```python
from build123d import *

# Parameters (mm, degrees)
SKETCH_1_W      = 10
SKETCH_1_H      = 40
SKETCH_1_W_2    = 40
SKETCH_1_H_2    = 10
EXTRUDE_1_DEPTH = 160


with BuildPart() as part:
    # Sketch 1 → Extrude 1 (new body)
    with BuildSketch(Plane.XY):
        Polygon((-25, 20), (-5, 20), (5, 20), (25, 20), (25, 30), (-25, 30), align=None)
        Rectangle(SKETCH_1_W, SKETCH_1_H)
        Polygon((5, -20), (-5, -20), (-30, -20), (-30, -30), (-20, -30), (20, -30), (30, -30), (30, -20), align=None)
        with Locations((0, -35)):
            Rectangle(SKETCH_1_W_2, SKETCH_1_H_2)
    extrude(amount=EXTRUDE_1_DEPTH)


solid = part.part
```
Could you check a few things on this model? Use its own coordinates, in mm. A direction names the side the tool comes from. Give positions to 0.01 mm unless a question says otherwise; leave off trailing zeros. Loops run counter-clockwise (first coordinate to the right, second up) from the corner with the lowest first, then second, coordinate; pieces in that order, holes last. Notation, with made-up numbers: (88.25, 79.5) - (106.25, 79.5) arc R25 cw to (106.25, 109.5) - close; hole circle Ø10 at (21.5, 9). An arc over 180 degrees is marked (long way). Use one line per item in the form item = value.
1. I want a section at D-D (y = 16). Please give me the cut outline in (x, z).
Response values:
outline = (-5, 0) - (5, 0) - (5, 160) - (-5, 160) - close
2. I need wall thicknesses on probe 1 along Y at (x, z) = (18, 16); probe 2 along Y at (x, z) = (23, 23); probe 3 along X at (y, z) = (-9, 140). Which ranges of each line are inside material? Lowest first, please.
Response values:
probe_1 = -40 to -20, 20 to 30
probe_2 = -30 to -20, 20 to 30
probe_3 = -5 to 5
3. I want a section at C-C (y = 23). Please give me the cut outline in (x, z).
Response values:
outline = (-25, 0) - (25, 0) - (25, 160) - (-25, 160) - close
4. Thinking about a two-plate mould opening in Y: for faces 1 (the face through (-15, 20, 79)), 2 (the face through (25, -30, 79)), 3 (the face through (0, 30, 79)), which applies, released by +Y, released by -Y, zero draft, split by the parting line, or undercut?
Response values:
face_1 = undercut
face_2 = released by -Y
face_3 = released by +Y
5. I want a section at B-B (z = 119). Please give me the cut outline in (x, y), and give its area (3 significant figures).
Response values:
outline = (-30, -30) - (-20, -30) - (-20, -40) - (20, -40) - (20, -30) - (30, -30) - (30, -20) - (5, -20) - (5, 20) - (25, 20) - (25, 30) - (-25, 30) - (-25, 20) - (-5, 20) - (-5, -20) - (-30, -20) - close
area = 1,900 mm²
6. On a 3-axis mill with a long thin cutter (end or side, diameter ignored), from which of +Z, -Z, +X, -X, +Y, -Y can I reach the whole of each face in a straight line? I mean faces 4 (the face through (-17, -20, 79)), 5 (the face through (15, 20, 79)), 6 (the face through (-20, -35, 79)), 7 (the face through (-25, 25, 79)), 8 (the face through (20, -35, 79)). Say none if no direction works.
Response values:
face_4 = +Z, -Z, -X
face_5 = +Z, -Z, +X
face_6 = +Z, -Z, -X, -Y
face_7 = +Z, -Z, -X, +Y
face_8 = +Z, -Z, +X, -Y
7. I want a section at A-A (x = -11). Please give me the cut outline in (y, z).
Response values:
outline = (-40, 0) - (-20, 0) - (-20, 160) - (-40, 160) - close; (20, 0) - (30, 0) - (30, 160) - (20, 160) - close
8. I'm going to push flat-ended pins straight in: pin 1 Ø5 at (y, z) = (10.5, 141.5) entering from -X; pin 2 Ø5 at (y, z) = (26, 52) entering from +X; pin 3 Ø3 at (y, z) = (-34.5, 115.5) entering from -X. Where does each tip first touch, or does it pass through?
Response values:
pin_1 = -5
pin_2 = 25
pin_3 = -20
